Input: dimensioned drawing with shaded views. Units: mm. Origin: part minimum x, y, z. A direction names the side the tool comes from. Give positions to 0.01 mm unless a question says otherwise; leave off trailing zeros. Order: outer loops, then holes, each group sorted by start corner. A loop starts at its lowest first (then second) coordinate and runs counter-clockwise, first axis right, second up. Notation, with made-up numbers: (10.5, 18) -> (24.5, 18) arc R10 cw to (24.5, 37) -> close; hole circle Ø3 at (-13.5, 72.25). An arc over 180 degrees is marked (long way). One line per question, with ' | ' between items. Start each with the question number.
(1) Ray query, L1, parallel to Y at x = 2.25, z = 3.5; L2, parallel to X at y = 6.5, z = 2.25; L3, parallel to X at y = 9.25, z = 7.75. Return the intervals inside material, ascending.
(2) Section A-A (x = 11). Return loops of the section in (y, z), then the cut area to 3 significant figures.
(3) Section B-B (x = 2.25). Return loops of the section in (y, z), then the cut area to 3 significant figures.
(4) Mould query, pull axis Y, two halves, no side actions, for the marked faces 5, 6, 7 and 8. Classes: +Y half, -Y half, draft (parallel to the pull), parting line (faces both ways), or undercut.
(5) Section C-C (z = 5.5). Return loops of the section in (x, y).
(6) First-contact query: pin 1 Ø0.9 at (x, y) = (13, 5) entering from +Z; pin 2 Ø6 at (y, z) = (4, 1.5) entering from +X; pin 3 Ø0.6 at (y, z) = (9.5, 5) entering from +X; pin 4 Ø1.5 at (y, z) = (6, 6) entering from -X. Flat tips, straight axial feed; report the tip coordinate or a pass-through.
(7) Set-up query: the marked faces 1, 2, 3 and 4. Return all of +Z, -Z, +X, -X, +Y, -Y with unobstructed straight access to the full face (end or side cutting, diameter ignored); none if empty.
(8) Section D-D (y = 4.25). Return loops of the section in (x, z), then the cut area to 3 significant figures.
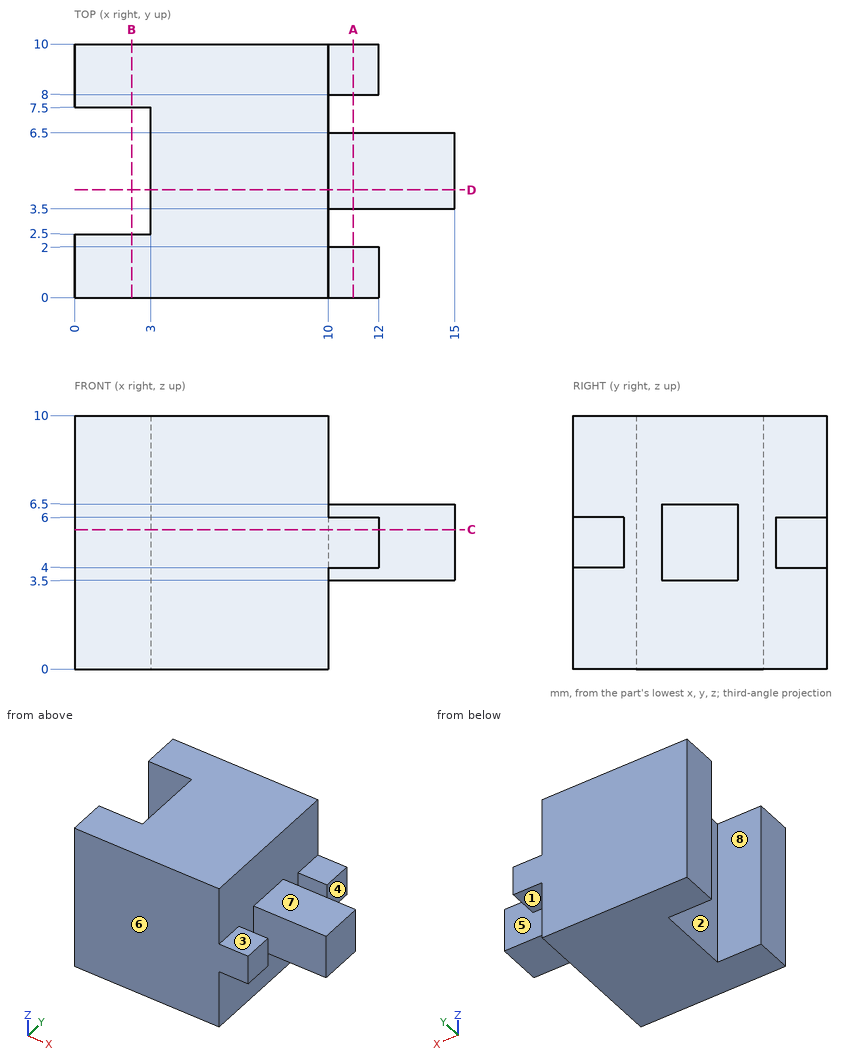
Response:
1) L1: y = 0 to 2.5, 7.5 to 10 | L2: x = 3 to 10 | L3: x = 0 to 10
2) outline: (0, 4) -> (2, 4) -> (2, 6) -> (0, 6) -> close; (3.5, 3.5) -> (6.5, 3.5) -> (6.5, 6.5) -> (3.5, 6.5) -> close; (8, 4) -> (10, 4) -> (10, 6) -> (8, 6) -> close | area: 17.0 mm^2
3) outline: (0, 0) -> (2.5, 0) -> (2.5, 10) -> (0, 10) -> close; (7.5, 0) -> (10, 0) -> (10, 10) -> (7.5, 10) -> close | area: 50.0 mm^2
4) face 5: undercut | face 6: -Y half | face 7: draft | face 8: undercut
5) outline: (0, 0) -> (12, 0) -> (12, 2) -> (10, 2) -> (10, 3.5) -> (15, 3.5) -> (15, 6.5) -> (10, 6.5) -> (10, 8) -> (12, 8) -> (12, 10) -> (0, 10) -> (0, 7.5) -> (3, 7.5) -> (3, 2.5) -> (0, 2.5) -> close
6) pin 1: stops at z = 6.5 | pin 2: stops at x = 15 | pin 3: stops at x = 12 | pin 4: stops at x = 3
7) face 1: -Z, +X, +Y | face 2: +Z, -Z, -X | face 3: +Z, +X, -Y | face 4: +Z, -Z, +X, +Y
8) outline: (3, 0) -> (10, 0) -> (10, 3.5) -> (15, 3.5) -> (15, 6.5) -> (10, 6.5) -> (10, 10) -> (3, 10) -> close | area: 85.0 mm^2
